Geometry: final body of the model. Coordinates: model frame, mm. Face numbers are marked on the shaded views. A direction names the side the tool comes from. Give positions to 0.01 mm unless a question says otherwise; leave off trailing zeros. Order: outer loops, then holes, each group sorted by start corner. A loop starts at its lowest first (then second) coordinate and runs counter-clockwise, first axis right, second up. Notation, with made-up numbers: (6.5, 25) -> (44.5, 25) arc R20 cw to (44.5, 64) -> close; hole circle Ø10 at (73.5, -23.5). An arc over 180 degrees is marked (long way). Write item = value, one per line.
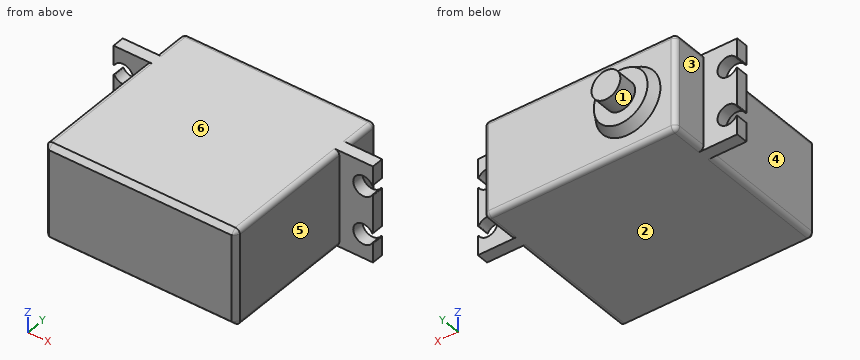
```python
from build123d import *

# Parameters (mm, degrees)
SKETCH1_W           = 40
SKETCH1_H           = 20
BOSS_EXTRUDE1_DEPTH = 28
SKETCH2_W           = 54
SKETCH2_H           = 20
BOSS_EXTRUDE2_DEPTH = 2.5
SKETCH3_W           = 40
SKETCH3_H           = 20
BOSS_EXTRUDE3_DEPTH = 7.5
SKETCH4_R           = 6.75
BOSS_EXTRUDE4_DEPTH = 2
SKETCH5_R           = 3
BOSS_EXTRUDE5_DEPTH = 4
FILLET1_R           = 1
CHAMFER1_SIZE       = 1
CHAMFER2_SIZE2      = 1.154700538
CHAMFER2_SIZE       = 2
SKETCH6_R           = 2.1
CUT_EXTRUDE1_DEPTH  = 60.491596045
FILLET2_R           = 0.1


with BuildPart() as part:
    # Sketch1 → Boss-Extrude1 (new body)
    with BuildSketch(Plane(origin=(0, 0, 0), x_dir=(1, 0, 0), z_dir=(0, 1, 0))):
        with Locations((20, 10)):
            Rectangle(SKETCH1_W, SKETCH1_H)
    extrude(amount=BOSS_EXTRUDE1_DEPTH)

    # Sketch2 → Boss-Extrude2 (add)
    with BuildSketch(Plane(origin=(0, 28, 0), x_dir=(1, 0, 0), z_dir=(0, 1, 0))):
        with Locations((20, 10)):
            Rectangle(SKETCH2_W, SKETCH2_H)
    extrude(amount=BOSS_EXTRUDE2_DEPTH)

    # Sketch3 → Boss-Extrude3 (add)
    with BuildSketch(Plane(origin=(0, 30.5, 0), x_dir=(1, 0, 0), z_dir=(0, 1, 0))):
        with Locations((20, 10)):
            Rectangle(SKETCH3_W, SKETCH3_H)
    extrude(amount=BOSS_EXTRUDE3_DEPTH)

    # Sketch4 → Boss-Extrude4 (add)
    with BuildSketch(Plane(origin=(0, 38, 0), x_dir=(1, 0, 0), z_dir=(0, 1, 0))):
        with Locations(Location((10, 10, 0), (0, 0, 270))):
            Circle(SKETCH4_R)
    extrude(amount=BOSS_EXTRUDE4_DEPTH)

    # Sketch5 → Boss-Extrude5 (add)
    with BuildSketch(Plane(origin=(0, 40, 0), x_dir=(1, 0, 0), z_dir=(0, 1, 0))):
        with Locations(Location((10, 10, 0), (0, 0, 270))):
            Circle(SKETCH5_R)
    extrude(amount=BOSS_EXTRUDE5_DEPTH)

    # Fillet1
    fillet1_edges = [part.edges().sort_by_distance(p)[0] for p in [
        (40, 14, -20),
        (40, 34.25, -20),
        (40, 34.25, 0),
        (40, 14, 0),
        (0, 34.25, 0),
        (0, 14, 0),
        (0, 14, -20),
        (0, 34.25, -20),
        (20, 38, -20),
        (40, 38, -10),
        (0, 38, -10),
        (20, 38, 0),
    ]]
    fillet(fillet1_edges, radius=FILLET1_R)

    # Chamfer1
    chamfer1_edges = [part.edges().sort_by_distance(p)[0] for p in [
        (20, 0, -20),
        (0, 0, -10),
        (40, 0, -10),
        (20, 0, 0),
        (0.292893219, 0, -19.707106781),
        (0.292893219, 0, -0.292893219),
        (39.707106781, 0, -0.292893219),
        (39.707106781, 0, -19.707106781),
    ]]
    chamfer(chamfer1_edges, length=CHAMFER1_SIZE)

    # Chamfer2
    chamfer2_edges = [part.edges().sort_by_distance(p)[0] for p in [
        (10, 40, -16.75),
    ]]
    chamfer2_side = [part.faces().sort_by_distance(p)[0] for p in [
        (10, 39.976905989, -16.75),
    ]]
    chamfer(chamfer2_edges, length=CHAMFER2_SIZE - 0.0001, length2=CHAMFER2_SIZE2 - 0.0001, reference=chamfer2_side[0])  # a hair under: the kernel refuses the full size

    # Sketch6 → Cut-Extrude1 (cut, through all)
    with BuildSketch(Plane(origin=(0, 30.5, 0), x_dir=(1, 0, 0), z_dir=(0, 1, 0))):
        with Locations((-5, 5)):
            Circle(SKETCH6_R)
        with Locations((-5, 15)):
            Circle(SKETCH6_R)
    cut_extrude1 = extrude(amount=-CUT_EXTRUDE1_DEPTH, mode=Mode.SUBTRACT)

    # Mirror2: Cut-Extrude1 across plane
    add(cut_extrude1.mirror(Plane.ZY.offset(-20)), mode=Mode.SUBTRACT)

    # Fillet2
    fillet2_edges = [part.edges().sort_by_distance(p)[0] for p in [
        (-7, 29.25, -4.359687576),
        (-7, 29.25, -5.640312424),
        (-7, 29.25, -15.640312424),
        (-7, 29.25, -14.359687576),
        (47, 29.25, -4.359687576),
        (47, 29.25, -5.640312424),
        (47, 29.25, -14.359687576),
        (47, 29.25, -15.640312424),
    ]]
    fillet(fillet2_edges, radius=FILLET2_R)


solid = part.part
```
1) Section query A-A (x = -5). Output: boundary loops of the cut face in (y, z).
Check sheet entries:
outline = (28, -20) -> (30.5, -20) -> (30.5, -17.1) -> (28, -17.1) -> close; (28, -12.9) -> (30.5, -12.9) -> (30.5, -7.1) -> (28, -7.1) -> close; (28, -2.9) -> (30.5, -2.9) -> (30.5, 0) -> (28, 0) -> close
2) First-contact query: P1, Ø12, axis at y = 19, z = -8, coming from the -X side; P2, Ø2.5, axis at x = 41.5, z = -14.5, coming from the +Y side; P3, Ø4, axis at x = 7.5, z = -3.5, coming from the +Y side; P4, Ø3.5, axis at x = -5, z = -15, coming from the +Y side. Flat tips, straight axial feed; report the tip coordinate or a pass-through.
Check sheet entries:
P1 = 0
P2 = 30.5
P3 = 40
P4 = through
3) Mould query, pull axis X, two halves, no side actions, for the marked faces 4, 5 and 6. Classes: +X half, -X half, draft (parallel to the pull), parting line (faces both ways), or undercut.
Check sheet entries:
face_4 = -X half
face_5 = +X half
face_6 = draft
4) Section query D-D (x = 35.5). Output: boundary loops of the cut face in (y, z).
Check sheet entries:
outline = (0, -19) -> (1, -20) -> (37, -20) arc R1 ccw to (38, -19) -> (38, -1) arc R1 ccw to (37, 0) -> (1, 0) -> (0, -1) -> close
5) Line query: line 1 (Z direction, x = -5, y = 29.65); line 2 (X direction, y = 8.5, z = -3.75); line 3 (Y direction, x = 32.5, z = -1.5). Output: solid intervals per line, ascending. Write a range as from..to.
Check sheet entries:
line_1 = -20..-17.1, -12.9..-7.1, -2.9..0
line_2 = 0..40
line_3 = 0..38
6) Reachability of the marked faces 1, 2 and 3 from +Z, -Z, +X, -X, +Y, -Y: full face, straight path, thin tool, end or side. Return the list, or none.
Check sheet entries:
face_1 = +Y
face_2 = -Z, +X, -X, +Y, -Y
face_3 = +Z, -Z, -X, +Y
7) Section query C-C (y = 5). Output: boundary loops of the cut face in (x, z), plus the area to 3 significant figures.
Check sheet entries:
outline = (0, -19) arc R1 ccw to (1, -20) -> (39, -20) arc R1 ccw to (40, -19) -> (40, -1) arc R1 ccw to (39, 0) -> (1, 0) arc R1 ccw to (0, -1) -> close
area = 799 mm²
